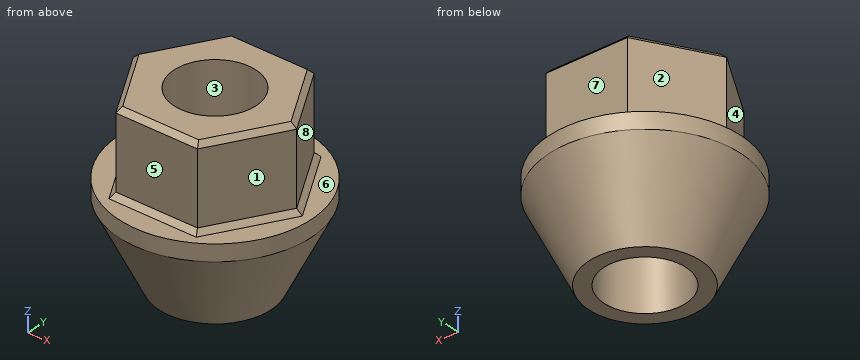
from build123d import *

# Parameters (mm, degrees)
EXTRUDE1_DEPTH     = 12.7
SKETCH3_R          = 14.869502809
EXTRUDE2_DEPTH     = 2.54
CHAMFER1_SIZE      = 0.762
CHAMFER2_SIZE      = 0.762
SKETCH5_R          = 14.869502809
EXTRUDE3_DEPTH     = 12.7
EXTRUDE3_TAPER     = 26
SKETCH4_R          = 6.35
CUT_EXTRUDE1_DEPTH = 28.9400001


with BuildPart() as part:
    # Sketch2 → Extrude1 (new body)
    with BuildSketch(Plane.XY):
        Polygon((12.673375262, 0), (6.336687631, 10.975464929), (-6.336687631, 10.975464929), (-12.673375262, 0), (-6.336687631, -10.975464929), (6.336687631, -10.975464929), align=None)
    extrude(amount=EXTRUDE1_DEPTH)

    # Sketch3 → Extrude2 (add)
    with BuildSketch(Plane(origin=(0, 0, 0), x_dir=(-1, 0, 0), z_dir=(0, 0, -1))):
        Circle(SKETCH3_R)
    extrude(amount=EXTRUDE2_DEPTH)

    # Chamfer1
    chamfer1_edges = [part.edges().sort_by_distance(p)[0] for p in [
        (0, -10.975464929, 0),
        (-9.505031447, -5.487732464, 0),
        (-9.505031447, 5.487732464, 0),
        (0, 10.975464929, 0),
        (9.505031447, 5.487732464, 0),
        (9.505031447, -5.487732464, 0),
    ]]
    chamfer(chamfer1_edges, length=CHAMFER1_SIZE)

    # Chamfer2
    chamfer2_edges = [part.edges().sort_by_distance(p)[0] for p in [
        (0, 10.975464929, 12.7),
        (-9.505031447, 5.487732464, 12.7),
        (-9.505031447, -5.487732464, 12.7),
        (0, -10.975464929, 12.7),
        (9.505031447, -5.487732464, 12.7),
        (9.505031447, 5.487732464, 12.7),
    ]]
    chamfer(chamfer2_edges, length=CHAMFER2_SIZE)

    # Sketch5 → Extrude3 (add)
    with BuildSketch(Plane(origin=(0, 0, -2.54), x_dir=(-1, 0, 0), z_dir=(0, 0, -1))):
        Circle(SKETCH5_R)
    extrude(amount=EXTRUDE3_DEPTH, taper=EXTRUDE3_TAPER)

    # Sketch4 → Cut-Extrude1 (cut, through all)
    with BuildSketch(Plane.XY.offset(12.7)):
        Circle(SKETCH4_R)
    extrude(amount=-CUT_EXTRUDE1_DEPTH, mode=Mode.SUBTRACT)


solid = part.part
For this review, take the finished solid that the model builds, in its own axes (mm). Face numbers are marked on the shaded views. A direction names the side the tool comes from. Round coordinates to 2 decimals unless told otherwise and drop trailing zeros. Order: outer loops, then holes, each group sorted by start corner. A loop starts at its lowest first (then second) coordinate and runs counter-clockwise, first axis right, second up. Notation, with made-up numbers: M 71.5,89 L 105.5,89 A26 ccw 105.5,122 Z; hole C -2.75,-5.75 d8. An arc over 180 degrees is marked long. Write each question's results on one line, items separated by ' | '. Start each with the question number.
1. To check wall thickness, follow L1, parallel to Y at x = 0, z = 6.25; L2, parallel to Y at x = 0, z = -2. State the ranges of each line that lie inside material, in increasing order. Write a range as [from, to].
2. Tool access review of the marked faces 4, 5, 6, 7 and 8: name each direction out of +Z, -Z, +X, -X, +Y, -Y from which nothing blocks a thin tool from reaching the whole face with its end or side.
3. Add section D-D (z = -12). State the section outline as (x, y) points.
4. Add section C-C (z = -4.5). State the section outline as (x, y) points, then the cut area to 3 significant figures.
5. Add section A-A (x = 0). State the section outline as (y, z) points.
6. Add section B-B (z = 8). State the section outline as (x, y) points, then the cut area to 3 significant figures.
7. Draft analysis for pull direction Y (two halves, no side actions). For the marked faces 1, 2 and 3, state which applies: pulls with the +Y half, pulls with the -Y half, needs draft (parallel to the pull), parting line crosses it, or undercut.
8. Clearance check with flat-ended pins moving along their axes: pin 1 Ø10 at (x, z) = (11, 2) entering from -Y; pin 2 Ø9 at (x, z) = (1, 9) entering from -Y; pin 3 Ø11.5 at (x, y) = (0, 0) entering from -Z; pin 4 Ø3.5 at (x, z) = (0.5, 6.5) entering from +Y. State where each tip first meets the part, or that it passes through.
Output values:
1) L1: [-10.98, -6.35], [6.35, 10.98] | L2: [-14.87, -6.35], [6.35, 14.87]
2) face 4: +Z, -X, -Y | face 5: +Z, +X, -X, -Y | face 6: +Z | face 7: +Z, +X, -X, +Y | face 8: +Z, +X, +Y
3) outline: C 0,0 d20.51; hole C 0,0 d12.7
4) outline: C 0,0 d27.83; hole C 0,0 d12.7 | area: 481 mm^2
5) outline: M -14.87,-2.54 L -8.68,-15.24 L -6.35,-15.24 L -6.35,12.7 L -10.21,12.7 L -10.98,11.94 L -10.98,0.76 L -11.74,0 L -14.87,0 Z; M 6.35,-15.24 L 8.68,-15.24 L 14.87,-2.54 L 14.87,0 L 11.74,0 L 10.98,0.76 L 10.98,11.94 L 10.21,12.7 L 6.35,12.7 Z
6) outline: M -12.67,0 L -6.34,-10.98 L 6.34,-10.98 L 12.67,0 L 6.34,10.98 L -6.34,10.98 Z; hole C 0,0 d12.7 | area: 291 mm^2
7) face 1: pulls with the -Y half | face 2: pulls with the +Y half | face 3: undercut
8) pin 1: y = -13.41 | pin 2: y = -10.98 | pin 3: through | pin 4: y = 10.98
